Job drawing, mm, ordinate dimensions from the low corner. One solid piece. Coordinates: 2 decimals unless noted, no trailing zeros. Write each loop counter-clockwise with the first axis right and the second up, starting at its lowest first coordinate (ties: lowest second). Pieces come first, ordered by that corner, then holes. Notation, with made-up numbers: M -5.75,58 L 11.25,58 A25 cw 11.25,84 Z; hole C -36,22.5 d8. An arc over 180 degrees is marked long. Answer as CSV lines item,"result". Start each with the question number.
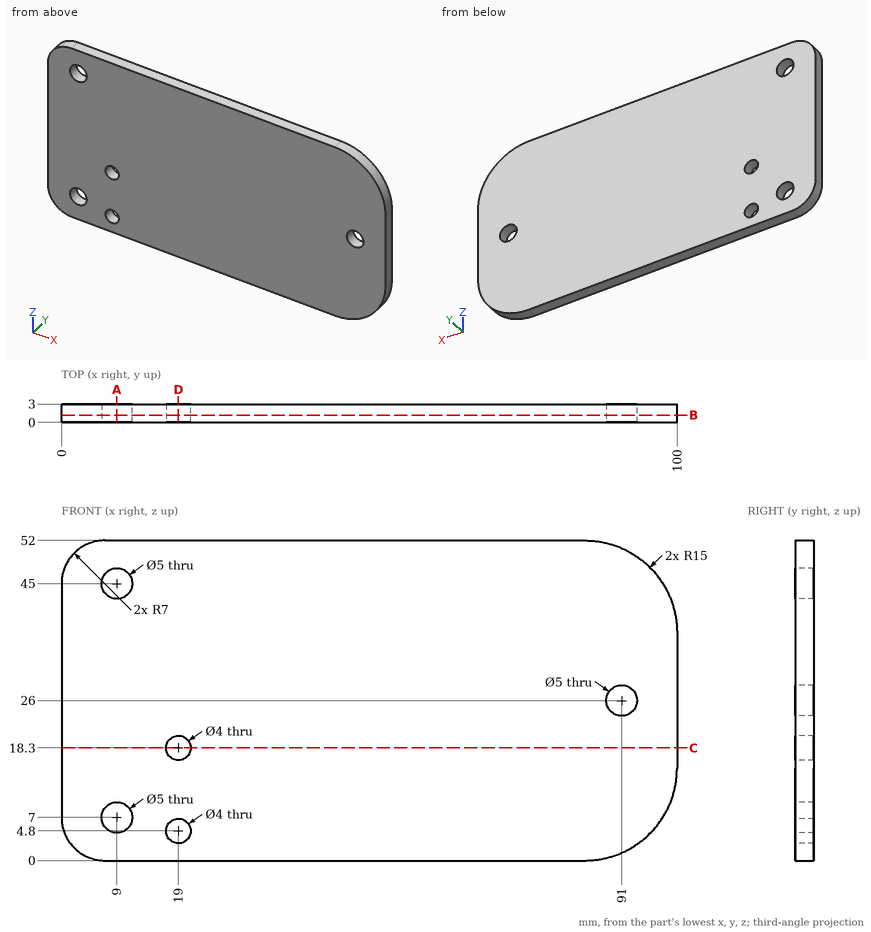
1) Probe L1, parallel to Z at x = 9, y = 1.35; L2, parallel to Z at x = 19, y = 1.1; L3, parallel to X at y = 1.05, z = 45. List the from-to ranges inside material, lowest first. Write a range as [from, to].
2) Pin check, flat tip, straight feed: P1, Ø8, axis at x = 9, z = 45, coming from the +Y side. Stop position of the tip, or through.
3) Band-saw the part on B-B, the plane y = 1.2. List the corners of the cut face in (x, z), plus the area to 3 significant figures.
4) Band-saw the part on C-C, the plane z = 18.3. List the corners of the cut face in (x, y).
5) Band-saw the part on A-A, the plane x = 9. List the corners of the cut face in (y, z).
6) Band-saw the part on D-D, the plane x = 19. List the corners of the cut face in (y, z).
Result sheet:
1,L1,"z = [0, 4.5], [9.5, 42.5], [47.5, 52]"
1,L2,"z = [0, 2.8], [6.8, 16.3], [20.3, 52]"
1,L3,"x = [0, 6.5], [11.5, 97.69]"
2,P1,"stops at y = 3"
3,outline,"M 0,7 A7 ccw 7,0 L 85,0 A15 ccw 100,15 L 100,37 A15 ccw 85,52 L 7,52 A7 ccw 0,45 Z; hole C 9,7 d5; hole C 9,45 d5; hole C 19,4.8 d4; hole C 19,18.3 d4; hole C 91,26 d5"
3,area,"5,000 mm²"
4,outline,"M 0,0 L 17,0 L 17,3 L 0,3 Z; M 21,0 L 100,0 L 100,3 L 21,3 Z"
5,outline,"M 0,0 L 3,0 L 3,4.5 L 0,4.5 Z; M 0,9.5 L 3,9.5 L 3,42.5 L 0,42.5 Z; M 0,47.5 L 3,47.5 L 3,52 L 0,52 Z"
6,outline,"M 0,0 L 3,0 L 3,2.8 L 0,2.8 Z; M 0,6.8 L 3,6.8 L 3,16.3 L 0,16.3 Z; M 0,20.3 L 3,20.3 L 3,52 L 0,52 Z"
